```python
from build123d import *

# Parameters (mm, degrees)
BOSS_EXTRUDE1_DEPTH = 3.2
CUT_EXTRUDE1_DEPTH  = 3
CUT_EXTRUDE2_START  = -3
CUT_EXTRUDE2_DEPTH  = 3


with BuildPart() as part:
    # Sketch1 → Boss-Extrude1 (new body)
    with BuildSketch(Plane.XY):
        with BuildLine():
            Line((-8.349125364, 0), (7.450874636, 0))
            ThreePointArc((7.450874636, 0), (-0.449125364, 7.386183646), (-8.349125364, 0))
        make_face()
    extrude(amount=BOSS_EXTRUDE1_DEPTH)

    # Sketch3 → Cut-Extrude1 (cut)
    with BuildSketch(Plane.XY.offset(3.2)):
        with BuildLine():
            Line((-3.19080338, 1.203425656), (-3.19080338, 1.560959579))
            Line((-3.19080338, 1.560959579), (-2.674178491, 1.739791271))
            Line((-2.674178491, 1.739791271), (-2.137683415, 1.560959579))
            Line((-2.137683415, 1.560959579), (-2.137683415, 1.203425656))
            Line((-2.137683415, 1.203425656), (1.239432686, 1.203425656))
            Line((1.239432686, 1.203425656), (1.239432686, 1.560959579))
            Line((1.239432686, 1.560959579), (1.775927763, 1.739791271))
            Line((1.775927763, 1.739791271), (2.292552651, 1.560959579))
            Line((2.292552651, 1.560959579), (2.292552651, 1.203425656))
            Line((2.292552651, 1.203425656), (6.281891371, 1.203425656))
            ThreePointArc((6.281891371, 1.203425656), (-0.47432937, 6.35784653), (-7.230550111, 1.203425656))
            Line((-7.230550111, 1.203425656), (-3.19080338, 1.203425656))
        make_face()
    extrude(amount=-CUT_EXTRUDE1_DEPTH, mode=Mode.SUBTRACT)

    # Sketch6 → Cut-Extrude2 (cut)
    with BuildSketch(Plane.XY.offset(3.2).offset(CUT_EXTRUDE2_START)):
        with BuildLine():
            Line((-3.866358844, 6.61080504), (-2.777388902, 5.968436276))
            ThreePointArc((-2.777388902, 5.968436276), (-5.071279367, 4.630051211), (-6.711633725, 2.54140437))
            Line((-6.711633725, 2.54140437), (-7.346913092, 3.355884027))
            ThreePointArc((-7.346913092, 3.355884027), (-5.857317606, 5.251403586), (-3.866358844, 6.61080504))
        make_face()
        with BuildLine():
            Line((5.778219706, 2.496322182), (6.448662363, 3.355884027))
            ThreePointArc((6.448662363, 3.355884027), (4.959066878, 5.251403586), (2.968108115, 6.61080504))
            Line((2.968108115, 6.61080504), (1.854961189, 5.954174597))
            ThreePointArc((1.854961189, 5.954174597), (4.155461155, 4.609729053), (5.778219706, 2.496322182))
        make_face()
    extrude(amount=CUT_EXTRUDE2_DEPTH, mode=Mode.SUBTRACT)


solid = part.part
```
Geometry check sheet. Reference: the model listing, model coordinates, mm. A direction names the side the tool comes from. Coordinates: 2 decimals unless noted, no trailing zeros. Write each loop counter-clockwise with the first axis right and the second up, starting at its lowest first coordinate (ties: lowest second). Pieces come first, ordered by that corner, then holes. Notation, with made-up numbers: M 84.5,-1 L 131.5,-1 A35 ccw 131.5,38 Z; hole C 40.5,27.5 d11. An arc over 180 degrees is marked long. Use one line per item in the form item = value. Start each with the question number.
1) Release check for a two-part mould opening along Y. For faces 5 (the flat face through (0, 1.203, 2)), 6 (the flat face through (-1, 0, 2)), 7 (the cylindrical face through (-0.424, 6.358, 1.721)), 8 (the flat face through (-7.02, 2.94, 1.68)) record: pulls with the +Y half, pulls with the -Y half, needs draft (parallel to the pull), parting line crosses it, or undercut.
2) Section check A-A on z = 0.8. Enter the section's corners in (x, y), and give its area (3 significant figures).
3) Section check D-D on x = -4.75. Enter the section's corners in (y, z), and give its area (3 significant figures).
4) Go/stop test with flat-tipped pins: pin 1 Ø1.5 at (x, z) = (-6, 2) entering from +Y; pin 2 Ø1.5 at (x, z) = (3.5, 1.5) entering from +Y; pin 3 Ø1.6 at (x, y) = (-1, 3.5) entering from +Z. Record where each tip stops, or that it passes through.
5) Set-up check for faces 1 (the flat face through (-5, 1.203, 2)), 2 (the flat face through (2.422, 6.289, 1.679)), 3 (the flat face through (-3.329, 6.294, 1.679)), 4 (the flat face through (6.11, 2.92, 1.68)): record each of +Z, -Z, +X, -X, +Y, -Y from which the full face is reachable in a straight line by a thin tool's end or side.
6) Thickness scan on probe 1 along Z at (x, y) = (-4.5, 5.5); probe 2 along Y at (x, z) = (-5.5, 3.05); probe 3 along X at (y, z) = (3, 0.65). Record the ranges inside material, lowest first. Write a range as from..to.
7) Section check B-B on x = -3. Enter the section's corners in (y, z), and give its area (3 significant figures).
8) Section check C-C on y = 2.25. Enter the section's corners in (x, z), and give its area (3 significant figures).
Responses:
q1.face_5 = undercut
q1.face_6 = pulls with the -Y half
q1.face_7 = undercut
q1.face_8 = pulls with the +Y half
q2.outline = M -8.35,0 L 7.45,0 A7.92 ccw 6.45,3.36 L 5.78,2.5 A7.01 cw 6.28,1.2 L 2.29,1.2 L 2.29,1.56 L 1.78,1.74 L 1.24,1.56 L 1.24,1.2 L -2.14,1.2 L -2.14,1.56 L -2.67,1.74 L -3.19,1.56 L -3.19,1.2 L -7.23,1.2 A7.01 cw -6.71,2.54 L -7.35,3.36 A7.92 ccw Z; M -3.87,6.61 L -2.78,5.97 A7.01 cw 1.86,5.96 L 2.97,6.61 A7.92 ccw Z
q2.area = 29.4 mm2
q3.outline = M 0,0 L 6.12,0 L 6.12,0.2 L 1.2,0.2 L 1.2,3.2 L 0,3.2 Z
q3.area = 4.83 mm2
q4.pin_1 = 2.59
q4.pin_2 = 6.71
q4.pin_3 = 0.2
q5.face_1 = +Z
q5.face_2 = +Z, +X
q5.face_3 = +Z, -X
q5.face_4 = +Z, +Y
q6.probe_1 = 0..0.2
q6.probe_2 = 0..1.2
q6.probe_3 = -7.54..-7.07, 6.17..6.64
q7.outline = M 0,0 L 6.96,0 L 6.96,3.2 L 6.1,3.2 L 6.1,0.2 L 1.63,0.2 L 1.63,3.2 L 0,3.2 Z
q7.area = 8.87 mm2
q8.outline = M -7.86,0 L 6.96,0 L 6.96,3.2 L 5.9,3.2 L 5.9,0.2 L -6.85,0.2 L -6.85,3.2 L -7.86,3.2 Z
q8.area = 9.18 mm2
